```python
from build123d import *

# Parameters (mm, degrees)
F1_DEPTH = 50


with BuildPart() as f1:
    # F0 (on Top) → F1 (new body)
    with BuildSketch(Plane.XY):
        Polygon((-3, 8), (-5, 10), (-10, 5), (-8, 3), (-5, 3), (-5, 5), (-3, 5), align=None)
        Polygon((5, 5), (3, 5), (-3, 5), (-5, 5), (-5, 3), (-5, -3), (-5, -5), (-3, -5), (3, -5), (5, -5), (5, -3), (5, 3), align=None)
        Polygon((10, 5), (5, 10), (3, 8), (3, 5), (5, 5), (5, 3), (8, 3), align=None)
        Polygon((5, -10), (10, -5), (8, -3), (5, -3), (5, -5), (3, -5), (3, -8), align=None)
        Polygon((-8, -3), (-10, -5), (-5, -10), (-3, -8), (-3, -5), (-5, -5), (-5, -3), align=None)
    extrude(amount=F1_DEPTH)


solid = f1.part
```
Check sheet for the modelled part. Datum: model origin and axes. Units: mm. A direction names the side the tool comes from. Round coordinates to 2 decimals unless told otherwise and drop trailing zeros. Loops run counter-clockwise (first coordinate to the right, second up) from the corner with the lowest first, then second, coordinate; pieces in that order, holes last. Notation, with made-up numbers: M -27.75,49 L -21.75,49 A28 ccw -21.75,76 Z; hole C 31,-30 d9. An arc over 180 degrees is marked long. Answer as a JSON object with one key per item and string values.
1. Section check D-D (x = 4.5). Record the boundary of the cut face in (y, z).
Reply:
{"outline": "M -9.5,0 L 9.5,0 L 9.5,50 L -9.5,50 Z"}
2. Mould release check, pull along Y, two halves, no side actions. Record for faces 1 (the flat face through (4, 9, 25)), 2 (the flat face through (-3, -7, 25)), 3 (the flat face through (7, -3, 25)): pulls with the +Y half, pulls with the -Y half, needs draft (parallel to the pull), parting line crosses it, or undercut.
Reply:
{"face 1": "pulls with the +Y half", "face 2": "needs draft", "face 3": "undercut"}
3. Section check A-A (y = -5.5). Record the boundary of the cut face in (x, z).
Reply:
{"outline": "M -9.5,0 L -3,0 L -3,50 L -9.5,50 Z; M 3,0 L 9.5,0 L 9.5,50 L 3,50 Z"}
4. Gauge pin test, flat ends, axial feed: P1, Ø6.5, axis at y = -1, z = 26, coming from the -X side; P2, Ø0.9, axis at x = -7, z = 26, coming from the +Y side; P3, Ø0.9, axis at y = -6, z = 16, coming from the -X side; P4, Ø2, axis at x = -1.5, y = -7, coming from the -Z side. Record the tip position at first contact, or that the pin passes through.
Reply:
{"P1": "stops at x = -9.25", "P2": "stops at y = 8.45", "P3": "stops at x = -9.45", "P4": "passes through"}
5. Scan lines: line 1 (X direction, y = 2.75, z = 14); line 2 (X direction, y = -6, z = 21). Record each from-to range of solid material in increasing order.
Reply:
{"line 1": "x = -5 to 5", "line 2": "x = -9 to -3, 3 to 9"}
6. Section check C-C (z = 13.5). Record the boundary of the cut face in (x, y).
Reply:
{"outline": "M -10,-5 L -5,-10 L -3,-8 L -3,-5 L 3,-5 L 3,-8 L 5,-10 L 10,-5 L 8,-3 L 5,-3 L 5,3 L 8,3 L 10,5 L 5,10 L 3,8 L 3,5 L -3,5 L -3,8 L -5,10 L -10,5 L -8,3 L -5,3 L -5,-3 L -8,-3 Z"}
7. Access from +Z, -Z, +X, -X, +Y, -Y to the whole of each face (thin tool, end or side, straight path). Record for faces 4 (the flat face through (3, 7, 25)), 5 (the flat face through (3, -6, 25)), 6 (the flat face through (9, -4, 25)), 7 (the flat face through (-5, 0, 25)).
Reply:
{"face 4": "+Z, -Z, +Y", "face 5": "+Z, -Z, -Y", "face 6": "+Z, -Z, +X", "face 7": "+Z, -Z, -X"}
8. Section check B-B (x = -6.75). Record the boundary of the cut face in (y, z).
Reply:
{"outline": "M -8.25,0 L -3,0 L -3,50 L -8.25,50 Z; M 3,0 L 8.25,0 L 8.25,50 L 3,50 Z"}
